Autodesk Inventor part; units mm, degrees
ref_plane "YZ Plane" through (0, 0, 0) normal (1, 0, 0) x (0, 1, 0)
ref_plane "XZ Plane" through (0, 0, 0) normal (0, 1, 0) x (-1, 0, 0)
ref_plane "XY Plane" through (0, 0, 0) normal (0, 0, 1) x (1, 0, 0)
sketch "Sketch1" plane through (0, 0, 0) normal (0, 1, 0) x (-1, 0, 0)
  line L0 (-5.75, 13.75) -> (5.75, 13.75)
  line L1 (5.75, 13.75) -> (5.75, -13.75)
  line L2 (5.75, -13.75) -> (-5.75, -13.75)
  line L3 (-5.75, -13.75) -> (-5.75, 13.75)
  line L4 (-5.75, 13.75) -> (5.75, -13.75) construction
  line L5 (5.75, 13.75) -> (-5.75, -13.75) construction
  line L6 (0, 8) -> (0, -8) construction
  point P0 (0, 0)
  point P1 (0, 0)
  dimension "d0" = 16
  dimension "d18" = 27.5
  dimension "d19" = 11.5
extrude "Extrusion1" add sketch "Sketch1" along normal blind 19
fillet "Fillet1" radius 5 2 edges at (5.75, 9.5, 13.75) (-5.75, 9.5, 13.75)
sketch "Sketch3" plane through (0, 19, 0) normal (0, 1, 0) x (1, 0, 0)
  line L0 (0, 7.25) -> (0, -8.75) construction
  line L1 (-5.75, 13.75) -> (-5.75, -8.75) construction
  line L2 (-0.75, -13.75) -> (0.75, -13.75)
  point P0 (0, 0)
  dimension "d7" = 16
  dimension "d8" = 5.75
  dimension "d9" = 5
hole "Hole1" at (0, 19, -7.25) at (0, 19, 8.75) direction (0, -1, 0) diameter 3.8 depth 8
sketch "Sketch4" plane through (-5.75, 0, -13.75) normal (-1, 0, 0) x (0, 0, 1)
  line L0 (27.5, 0) -> (27.5, 19)
  point P0 (13.75, 0)
  point P1 (3.85, 4.1)
  dimension "d17" = 23.65
  dimension "d20" = 4.1
hole "Hole2" at (-5.75, 4.1, -9.9) direction (1, 0, 0) diameter 5.5 end through all
sketch "Sketch5" plane through (0, 19, 0) normal (0, 1, 0) x (1, 0, 0)
  line L0 (5.75, 13.75) -> (-5.75, 13.75) construction
  line L1 (-5.75, 13.75) -> (5.75, 13.75)
  line L2 (5.75, 13.75) -> (5.75, 24.25)
  line L3 (5.75, 24.25) -> (-5.75, 24.25)
  line L4 (-5.75, 24.25) -> (-5.75, 13.75)
  line L5 (-0.75, -13.75) -> (0.75, -13.75)
  point P0 (0, 0)
  point P1 (0, -13.75)
  dimension "d28" = 38
extrude "Extrusion2" add sketch "Sketch5" against normal up to surface (19 mm away)
sketch "Sketch7" plane through (0, 19, 0) normal (0, 1, 0) x (1, 0, 0)
  circle A0 centre (0, 7.25) radius 1.9 construction
  circle A1 centre (0, -8.75) radius 1.9 construction
  point P0 (0, 0)
  point P1 (-1.75, 17.25)
  dimension "d31" = 1.75
  dimension "d32" = 10
hole "Hole3" at (-1.75, 19, -17.25) direction (0, -1, 0) diameter 5.5 depth 8
sketch "Sketch9" plane through (0, 0, 0) normal (0, -1, 0) x (1, 0, 0)
  line L0 (5.75, 8.75) -> (5.75, -24.25) construction
  line L1 (-5.75, -24.25) -> (-5.75, 8.75) construction
  line L2 (5.75, -24.25) -> (-5.75, -24.25)
  line L3 (-5.75, -24.25) -> (-5.75, -12.25)
  line L4 (-5.75, -12.25) -> (5.75, -12.25)
  line L5 (5.75, -12.25) -> (5.75, -24.25)
  point P0 (0, 0)
  dimension "d47" = 12
extrude "Extrusion3" add sketch "Sketch9" along normal blind 21
chamfer "Chamfer1" distance 10 angle 45 1 edges at (0, 0, -12.25)
sketch "Sketch10" plane through (0, -21, 0) normal (0, -1, 0) x (1, 0, 0)
  circle A0 centre (-1.75, -17.25) radius 2.75 construction
  point P0 (0, 0)
hole "Hole5" at (-1.75, -21, -17.25) direction (0, 1, 0) diameter 5.5 depth 8
fillet "Fillet2" radius 2 4 edges at (-5.75, -1, -24.25) (5.75, -1, -24.25) (-5.75, -15.5, -12.25) (5.75, -15.5, -12.25)
properties part number "CH_01_0040_kradex_mount_2"
Here's how the part is built. I have some questions about the finished solid (model axes, mm). A direction names the side the tool comes from. Coordinates: 2 decimals unless noted, no trailing zeros. Write each loop counter-clockwise with the first axis right and the second up, starting at its lowest first coordinate (ties: lowest second). Pieces come first, ordered by that corner, then holes.
Item 1: I want a section at C-C on x = 0. Write out the boundary of the cut face in (y, z), and give its area (3 significant figures).
Item 2: On a 3-axis mill with a long thin cutter (end or side, diameter ignored), from which of +Z, -Z, +X, -X, +Y, -Y can I reach the whole of each face in a straight line? I mean faces 1 (the flat face through (0, 11, -7)), 2 (the flat face through (-5.75, 4, -7)), 3 (the flat face through (0, -1, -24.25)), 4 (the cylindrical face through (-5.15, -15.58, -12.82)), 5 (the cylindrical face through (5.18, -15.58, -12.85)). Say none if no direction works.
Item 3: If we mould it in two halves opening along Z, with no side actions, what happens to faces 6 (the flat face through (-2, -13, -17)), 7 (the cylindrical face through (-4.32, 9.63, 12.25)), 8 (the flat face through (0, 0, 6))? For each: +Z half, -Z half, draft (parallel to the pull), parting line (faces both ways), or undercut.
Item 4: I want a section at A-A on y = 4.1. Write out the boundary of the cut face in (x, z), and give its area (3 significant figures).
Item 5: If I drill on line 1 (X direction, y = 13, z = -17); line 2 (Z direction, x = 0, y = 15.75); line 3 (Z direction, x = 0, y = -16.5), over which ranges is the centre line in solid material (lowest first)?
Item 6: I want a section at B-B on z = -9.9. Write out the boundary of the cut face in (x, y), and give its area (3 significant figures).
Item 7: Will these pins go through, and if not, where does the flat tip stop? pin 1 (5 mm diameter, centred on x = 0, z = 8.75, fed in from -Y); pin 2 (4.5 mm diameter, centred on y = 4.1, z = -9.9, fed in from -X); pin 3 (4.5 mm diameter, centred on x = -2, z = -17, fed in from -Y); pin 4 (1.1 mm diameter, centred on x = -1, z = -8, fed in from +Y).
Item 8: I want a section at D-D on y = 14. Write out the boundary of the cut face in (x, z).
Findings below:
1. outline: (-21, -24.25) - (19, -24.25) - (19, -19.37) - (11, -19.37) - (11, -15.13) - (19, -15.13) - (19, -9.15) - (11, -9.15) - (11, -5.35) - (19, -5.35) - (19, 6.85) - (11, 6.85) - (11, 10.65) - (19, 10.65) - (19, 13.75) - (0, 13.75) - (0, -2.25) - (-10, -12.25) - (-21, -12.25) - (-21, -15.13) - (-13, -15.13) - (-13, -19.37) - (-21, -19.37) - close; hole circle Ø5.5 at (4.1, -9.9)
1. area: 872 mm2
2. face 1: +Y
2. face 2: +Z, -Z, -X, +Y, -Y
2. face 3: -Z, +X, -X, +Y, -Y
2. face 4: +Z, -X, -Y
2. face 5: +Z, +X, -Y
3. face 6: undercut
3. face 7: +Z half
3. face 8: draft
4. outline: (-5.75, -22.25) arc R2 ccw to (-3.75, -24.25) - (3.75, -24.25) arc R2 ccw to (5.75, -22.25) - (5.75, -12.65) - (-5.75, -12.65) - close; (-5.75, -7.15) - (5.75, -7.15) - (5.75, 8.75) arc R5 ccw to (0.75, 13.75) - (-0.75, 13.75) arc R5 ccw to (-5.75, 8.75) - close
4. area: 361 mm2
5. line 1: x = -5.75 to -4.49, 0.99 to 5.75
5. line 2: z = -24.25 to -19.37, -15.13 to -9.15, -5.35 to 6.85, 10.65 to 13.75
5. line 3: z = -24.25 to -19.37, -15.13 to -12.25
6. outline: (-5.75, -7.65) - (5.75, -7.65) - (5.75, 1.35) - (-5.75, 1.35) - close; (-5.75, 6.85) - (5.75, 6.85) - (5.75, 19) - (-5.75, 19) - close
6. area: 243 mm2
7. pin 1: stops at y = 0
7. pin 2: passes through
7. pin 3: stops at y = -13
7. pin 4: stops at y = 11
8. outline: (-5.75, -22.25) arc R2 ccw to (-3.75, -24.25) - (3.75, -24.25) arc R2 ccw to (5.75, -22.25) - (5.75, 8.75) arc R5 ccw to (0.75, 13.75) - (-0.75, 13.75) arc R5 ccw to (-5.75, 8.75) - close; hole circle Ø5.5 at (-1.75, -17.25); hole circle Ø3.8 at (0, -7.25); hole circle Ø3.8 at (0, 8.75)
